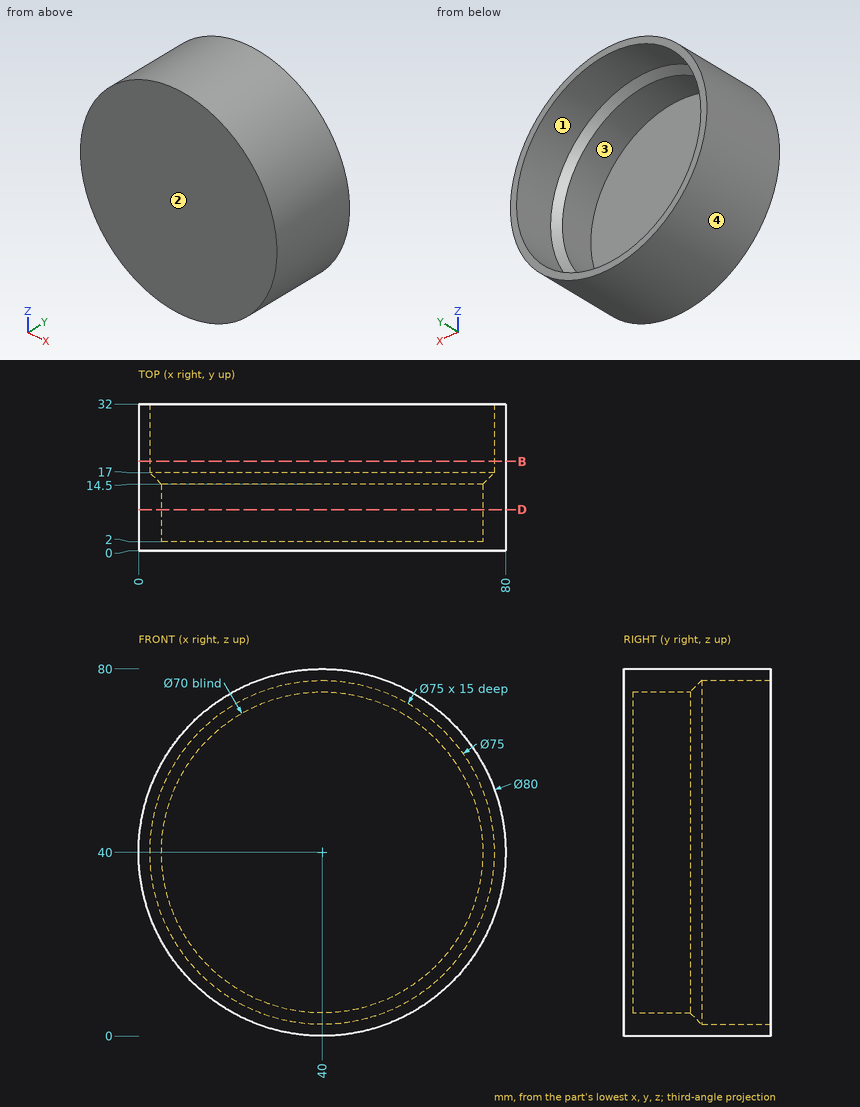
Drawing for the job (mm, zero at the part's lowest x, y, z). Round coordinates to 2 decimals unless told otherwise and drop trailing zeros. Order: outer loops, then holes, each group sorted by start corner. A loop starts at its lowest first (then second) coordinate and runs counter-clockwise, first axis right, second up. Notation, with made-up numbers: M 82,49.5 L 113,49.5 A23 ccw 113,67.5 Z; hole C -14,13.25 d7. An arc over 180 degrees is marked long. Use one line per item in the form item = value.
Q1. Flat gauge pins, fed straight in: P1, Ø2, axis at x = 32.5, z = 12.5, coming from the +Y side; P2, Ø12, axis at y = 7.5, z = 68.5, coming from the -X side; P3, Ø8, axis at y = 10, z = 46.5, coming from the -X side. Where does each tip first touch, or does it go through?
Recorded:
P1 = 2
P2 = 6.93
P3 = 0.08
Q2. Saw through at D-D on y = 9. Give the cut face in (x, z), then the cut area to 3 significant figures.
Recorded:
outline = C 40,40 d80; hole C 40,40 d70
area = 1,180 mm^2
Q3. Probe L1, parallel to X at y = 28.25, z = 40; L2, parallel to X at y = 8.5, z = 40; L3, parallel to Y at x = 63, z = 45. List the from-to ranges inside material, lowest first.
Recorded:
L1 = 0 to 2.5, 77.5 to 80
L2 = 0 to 5, 75 to 80
L3 = 0 to 2
Q4. Saw through at B-B on y = 19.5. Give the cut face in (x, z).
Recorded:
outline = C 40,40 d80; hole C 40,40 d75
Q5. Two-plate mould, pull along X, no slides. Class the marked faces 1, 2, 3 and 4: +X half, -X half, draft (parallel to the pull), parting line (faces both ways), or undercut.
Recorded:
face_1 = undercut
face_2 = draft
face_3 = undercut
face_4 = parting line
